Could you check a few things on this model? Use its own coordinates, in mm. Face numbers are marked on the shaded views. Give positions to 0.01 mm unless a question says otherwise; leave off trailing zeros. Loops run counter-clockwise (first coordinate to the right, second up) from the corner with the lowest first, then second, coordinate; pieces in that order, holes last. Notation, with made-up numbers: (-4, 12.5) -> (35, 12.5) arc R18 cw to (35, 42.5) -> close; hole circle Ø6 at (50, -37.75). An arc over 180 degrees is marked (long way). Write item = value, one per line. Start each with the question number.
1) I need wall thicknesses on probe 1 along Z at (x, y) = (-93, -116); probe 2 along X at (y, z) = (-287.5, -35); probe 3 along X at (y, z) = (-116.5, -21.5). Which ranges of each line are inside material? Lowest first, please. Write a range as from..to.
2) I want a section at A-A (z = -33.5). List the corners of the cut face in (x, y) for me, and give its area (3 significant figures).
3) I want a section at C-C (x = -95.5). List the corners of the cut face in (y, z) for me, and give its area (3 significant figures).
4) If we mould it in two halves opening along X, with no side actions, what happens to the marked faces 1, 2 and 3? For each: +X half, -X half, draft (parallel to the pull), parting line (faces both ways), or undercut.
5) I want a section at B-B (y = -49.5). List the corners of the cut face in (x, z) for me.
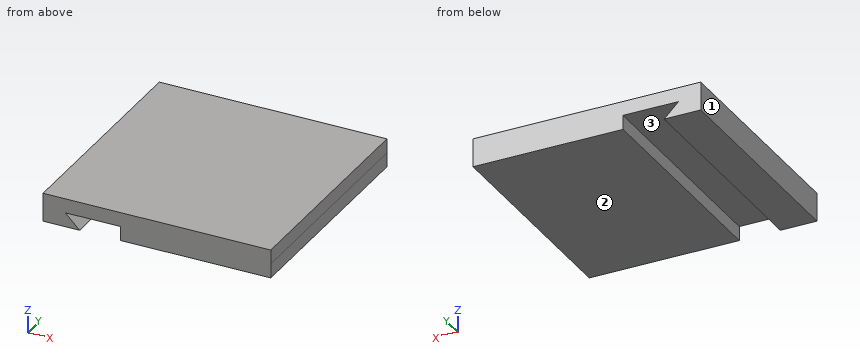
from build123d import *

# Parameters (mm, degrees)
F0_W     = 200.770747
F0_H     = 19.05
F1_DEPTH = 304.8


with BuildPart() as f1:
    # F0 (on Front) → F1 (new body)
    with BuildSketch(Plane.XZ):
        Polygon((-119.097248, -19.97675), (-148.705989, -19.97675), (-148.705989, -39.02675), (-99.606508, -39.02675), align=None)
        Polygon((156.094011, -0.92675), (-148.705989, -0.92675), (-148.705989, -19.97675), (-119.097248, -19.97675), (-44.676736, -19.97675), (156.094011, -19.97675), align=None)
        with Locations((55.708637, -29.50175)):
            Rectangle(F0_W, F0_H)
    extrude(amount=F1_DEPTH)


solid = f1.part
Answer list:
q1.probe_1 = -19.98..-0.93
q1.probe_2 = -148.71..-103.73, -44.68..156.09
q1.probe_3 = -148.71..-117.54, -44.68..156.09
q2.outline = (-148.71, -304.8) -> (-105.26, -304.8) -> (-105.26, 0) -> (-148.71, 0) -> close; (-44.68, -304.8) -> (156.09, -304.8) -> (156.09, 0) -> (-44.68, 0) -> close
q2.area = 74,400 mm^2
q3.outline = (-304.8, -19.98) -> (0, -19.98) -> (0, -0.93) -> (-304.8, -0.93) -> close
q3.area = 5,810 mm^2
q4.face_1 = -X half
q4.face_2 = draft
q4.face_3 = undercut
q5.outline = (-148.71, -39.03) -> (-99.61, -39.03) -> (-119.1, -19.98) -> (-44.68, -19.98) -> (-44.68, -39.03) -> (156.09, -39.03) -> (156.09, -0.93) -> (-148.71, -0.93) -> close
